```python
from build123d import *

# Parameters (mm, degrees)
F0_R     = 9.5
F0_R_2   = 2.525
F1_DEPTH = 5
F2_SIZE  = 0.1
F3_R     = 1
F4_DEPTH = 5.001
F5_SIZE  = 0.3


with BuildPart() as f1:
    # F0 (on Top) → F1 (new body)
    with BuildSketch(Plane.XY):
        Circle(F0_R)
        Circle(F0_R_2, mode=Mode.SUBTRACT)
    extrude(amount=F1_DEPTH)

    # F2
    f2_edges = [f1.edges().sort_by_distance(p)[0] for p in [
        (-9.5, 0, 5),
        (-9.5, 0, 0),
        (-2.525, 0, 5),
        (-2.525, 0, 0),
    ]]
    chamfer(f2_edges, length=F2_SIZE)

    # F3 (on face) → F4 (cut, through all)
    with BuildSketch(Plane.XY.offset(5)):
        with Locations((0, 6)):
            Circle(F3_R)
        with Locations((-6, 0)):
            Circle(F3_R)
        with Locations((0, -6)):
            Circle(F3_R)
        with Locations((6, 0)):
            Circle(F3_R)
    extrude(amount=-F4_DEPTH, mode=Mode.SUBTRACT)

    # F5
    f5_edges = [f1.edges().sort_by_distance(p)[0] for p in [
        (-1, 6, 5),
        (5, 0, 5),
        (-1, -6, 5),
        (-7, 0, 5),
        (-7, 0, 0),
        (-1, 6, 0),
        (5, 0, 0),
        (-1, -6, 0),
    ]]
    chamfer(f5_edges, length=F5_SIZE)


solid = f1.part
```
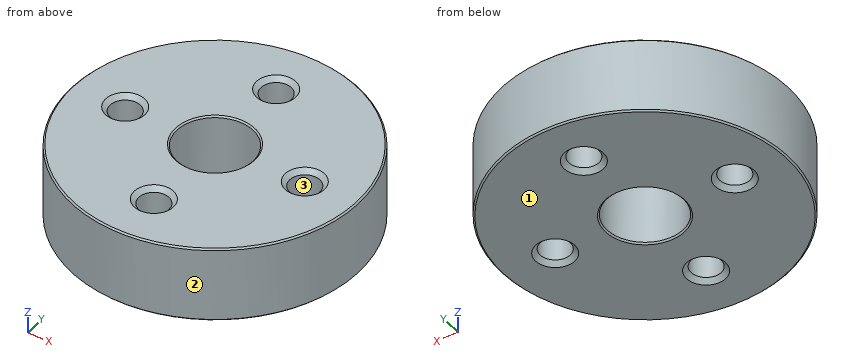
CAD build for the part. Positions are in the model's coordinates, mm. Face numbers are marked on the shaded views. Round coordinates to 2 decimals unless told otherwise and drop trailing zeros. Write each loop counter-clockwise with the first axis right and the second up, starting at its lowest first coordinate (ties: lowest second). Pieces come first, ordered by that corner, then holes.
Item 1: Band-saw the part on A-A on x = 0. Give the number of separate pieces and of enclosed holes in the cut face, then the cut area to 4 significant figures.
Filled in:
separate pieces: 4
enclosed holes: 0
area: 49.35 mm2
Item 2: Mould opens along Y. For the marked faces 1, 2 and 3 say: released by +Y, released by -Y, zero draft, split by the parting line, or undercut.
Filled in:
face 1: zero draft
face 2: split by the parting line
face 3: undercut
Item 3: Drop flat-ended pins along their axis: pin 1 Ø1 at (x, z) = (-7, 1) entering from +Y; pin 2 Ø3 at (y, z) = (6, 2.5) entering from +X; pin 3 Ø2.5 at (x, y) = (0, 6) entering from +Z. Give the stop position or say it passes through.
Filled in:
pin 1: stops at y = 6.93
pin 2: stops at x = 8.37
pin 3: stops at z = 4.95
Item 4: Band-saw the part on C-C on z = 1.55. Write the cut outline in (x, y) (3 decimals).
Filled in:
outline: circle Ø19 at (0, 0); hole circle Ø2 at (-6, 0); hole circle Ø5.05 at (0, 0); hole circle Ø2 at (0, -6); hole circle Ø2 at (0, 6); hole circle Ø2 at (6, 0)
Item 5: Drill centre lines: L1, parallel to Y at x = 0, z = 1.5 (3 decimals); L2, parallel to X at y = 6.25, z = 0.75; L3, parallel to Y at x = 5.75, z = 2.1. Where is each one in solid material? Low to high.
Filled in:
L1: y = -9.5 to -7, -5 to -2.525, 2.525 to 5, 7 to 9.5
L2: x = -7.15 to -0.97, 0.97 to 7.15
L3: y = -7.56 to -0.97, 0.97 to 7.56
